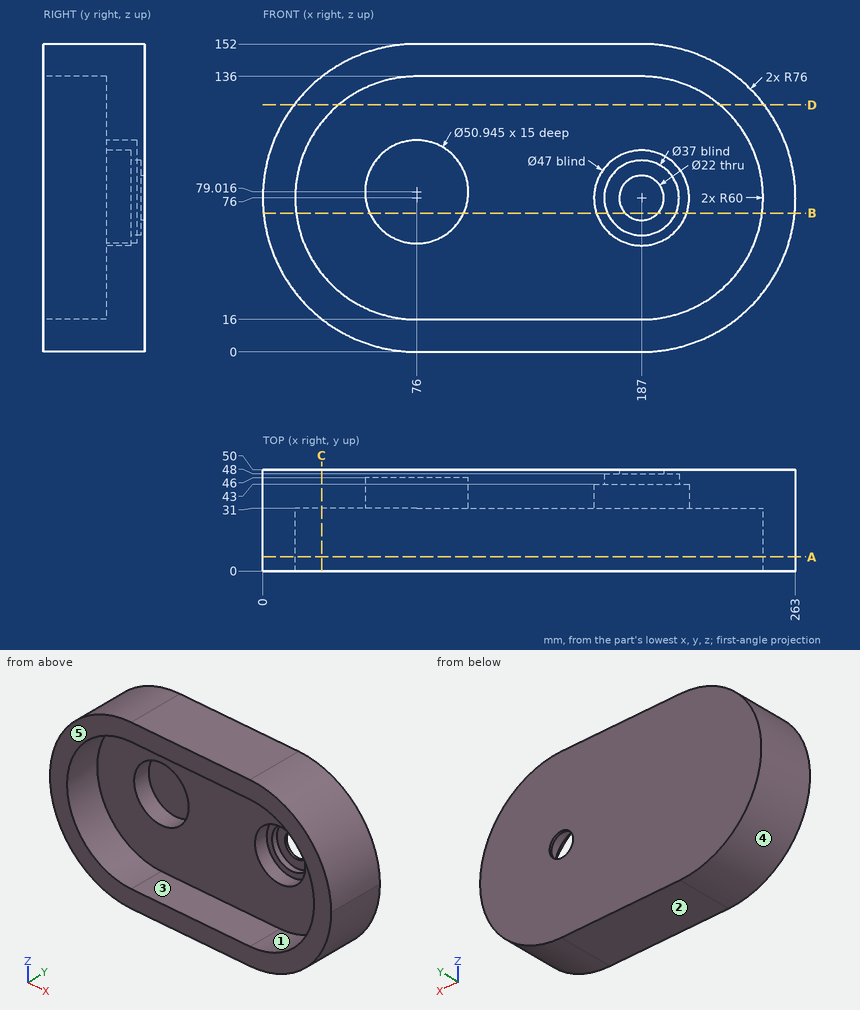
Here's the drawing with two shaded views (mm, measured from the low corner). I have some questions. A direction names the side the tool comes from. Coordinates: 2 decimals unless noted, no trailing zeros. Order: outer loops, then holes, each group sorted by start corner. A loop starts at its lowest first (then second) coordinate and runs counter-clockwise, first axis right, second up. Notation, with made-up numbers: (5.25, -0.75) - (47.25, -0.75) arc R12 cw to (47.25, 5.25) - close; hole circle Ø10 at (0, 40.5). An arc over 180 degrees is marked (long way). Answer in a Markdown table with one row per item. Add a question column.
(1) Will these pins go through, and if not, where does the flat tip stop? pin 1 (1 mm diameter, centred on y = 12.5, z = 30.5, fed in from +X) (1 decimal); pin 2 (1 mm diameter, centred on y = 14, z = 75, fed in from -X); pin 3 (6 mm diameter, centred on y = 40, z = 82.5, fed in from -X); pin 4 (13 mm diameter, centred on x = 187, z = 76, fed in from +Y).
(2) On a 3-axis mill with a long thin cutter (end or side, diameter ignored), from which of +Z, -Z, +X, -X, +Y, -Y can I reach the whole of each face in a straight line? I mean the marked faces 1 and 2. Say none if no direction works.
(3) If we section it at C-C, the plane x = 29: Please give me the cut outline in (y, z) (1 decimal), then the cut area to 3 significant figures.
(4) If we section it at B-B, the plane z = 68.5: Please give me the cut outline in (x, y).
(5) I need wall thicknesses on L1, parallel to Z at x = 187, y = 45.15; L2, parallel to Z at x = 187, y = 49; L3, parallel to X at y = 46.15, z = 76. Which ranges of each line are inside material? Lowest first, please.
(6) If we mould it in two halves opening along X, with no side actions, what happens to the marked faces 3, 4 and 5? For each: released by +X, released by -X, zero draft, split by the parting line, or undercut.
(7) If we section it at D-D, the plane z = 122: Please give me the cut outline in (x, y).
(8) If we section it at A-A, the plane y = 7: Please give me the cut outline in (x, z).
Results are:
| question | item | result |
|---|---|---|
| 1 | pin 1 | stops at x = 248.2 |
| 1 | pin 2 | stops at x = 0 |
| 1 | pin 3 | stops at x = 0.08 |
| 1 | pin 4 | passes through |
| 2 | face 1 | -Y |
| 2 | face 2 | -Z, +X, -X, +Y, -Y |
| 3 | outline | (0, 16.3) - (50, 16.3) - (50, 135.7) - (0, 135.7) - (0, 113.3) - (31, 113.3) - (31, 38.7) - (0, 38.7) - close |
| 3 | area | 3,660 mm2 |
| 4 | outline | (0.37, 0) - (16.47, 0) - (16.47, 31) - (52.8, 31) - (52.8, 46) - (99.2, 46) - (99.2, 31) - (164.73, 31) - (164.73, 43) - (170.09, 43) - (170.09, 48) - (178.95, 48) - (178.95, 50) - (0.37, 50) - close; (195.05, 48) - (203.91, 48) - (203.91, 43) - (209.27, 43) - (209.27, 31) - (246.53, 31) - (246.53, 0) - (262.63, 0) - (262.63, 50) - (195.05, 50) - close |
| 5 | L1 | z = 0 to 57.5, 94.5 to 152 |
| 5 | L2 | z = 0 to 65, 87 to 152 |
| 5 | L3 | x = 0 to 168.5, 205.5 to 263 |
| 6 | face 3 | undercut |
| 6 | face 4 | released by -X |
| 6 | face 5 | zero draft |
| 7 | outline | (15.5, 0) - (37.48, 0) - (37.48, 31) - (225.52, 31) - (225.52, 0) - (247.5, 0) - (247.5, 50) - (15.5, 50) - close |
| 8 | outline | (76, 0) - (187, 0) arc R76 ccw to (187, 152) - (76, 152) arc R76 ccw to start; hole (76, 16) - (187, 16) arc R60 ccw to (187, 136) - (76, 136) arc R60 ccw to start |
